Autodesk Inventor part; units mm, degrees
ref_plane "YZ Plane" through (0, 0, 0) normal (1, 0, 0) x (0, 1, 0)
ref_plane "XZ Plane" through (0, 0, 0) normal (0, 1, 0) x (-1, 0, 0)
ref_plane "XY Plane" through (0, 0, 0) normal (0, 0, 1) x (1, 0, 0)
sketch "Sketch1" plane through (0, 0, 0) normal (0, 1, 0) x (-1, 0, 0)
  line L0 (374.9202, -9.4574) -> (324.1202, -9.4574)
  line L1 (324.1202, -9.4574) -> (324.1202, -263.4574)
  line L2 (324.1202, -263.4574) -> (374.9202, -263.4574)
  line L3 (374.9202, -263.4574) -> (374.9202, -9.4574)
  point P0 (0, 0)
  dimension "d0" = 254
  dimension "d1" = 50.8
extrude "Extrusion1" add sketch "Sketch1" along normal blind 2.9972
sketch "Sketch2" plane through (0, 2.9972, 0) normal (0, 1, 0) x (1, 0, 0)
  line L0 (-336.8202, 206.3074) -> (-362.2202, 206.3074) construction
  line L1 (-362.2202, 206.3074) -> (-362.2202, 250.7574) construction
  line L2 (-362.2202, 250.7574) -> (-336.8202, 250.7574) construction
  line L3 (-336.8202, 250.7574) -> (-336.8202, 206.3074) construction
  line L4 (-336.8202, 206.3074) -> (-362.2202, 250.7574) construction
  line L5 (-362.2202, 206.3074) -> (-336.8202, 250.7574) construction
  line L6 (-324.1202, 263.4574) -> (-374.9202, 263.4574)
  line L7 (-349.5202, 228.5324) -> (-349.5202, 263.4574) construction
  circle A0 centre (-362.2202, 250.7574) radius 2.1828
  circle A1 centre (-336.8202, 250.7574) radius 2.1828
  circle A2 centre (-336.8202, 206.3074) radius 2.1828
  circle A3 centre (-362.2202, 206.3074) radius 2.1828
  point P0 (0, 0)
  dimension "d4" = 25.4
  dimension "d5" = 44.45
  dimension "d6" = 12.7
  dimension "d7" = 4.3656
extrude "Extrusion2" cut sketch "Sketch2" against normal through all
properties part number "10x2 Lexan" material "Polycarbonate, Clear"
Here's how the part is built. I have some questions about the finished solid (model axes, mm). Coordinates: 2 decimals unless noted, no trailing zeros. Answer as CSV lines item,"result". Start each with the question number.
1. We'd pull the mould along Z, two halves only. Please class faces 1 (the cylindrical face through (-335.65, 1.52, -252.6)), 2 (the flat face through (-349, 0, -135)): released by +Z, released by -Z, zero draft, split by the parting line, or undercut.
2. For pin 1 (1.5 mm diameter, centred on x = -340.5, z = -217.5, fed in from -Y); pin 2 (2.5 mm diameter, centred on x = -336.82, z = -250.76, fed in from -Y), each with a flat end and sliding along its axis, tell me the tip position at first contact or that it passes through.
3. I need wall thicknesses on line 1 (Z direction, x = -362.5, y = 2.4); line 2 (Z direction, x = -335.5, y = 1.65). Which ranges of each line are inside material? Lowest first, please. Write a range as [from, to].
Recorded:
1,face 1,"undercut"
1,face 2,"zero draft"
2,pin 1,"stops at y = 0"
2,pin 2,"passes through"
3,line 1,"z = [-263.46, -252.92], [-248.59, -208.47], [-204.14, -9.46]"
3,line 2,"z = [-263.46, -252.5], [-249.02, -208.05], [-204.57, -9.46]"
